Autodesk Inventor part; units mm, degrees
ref_plane "YZ Plane" through (0, 0, 0) normal (1, 0, 0) x (0, 1, 0)
ref_plane "XZ Plane" through (0, 0, 0) normal (0, 1, 0) x (-1, 0, 0)
ref_plane "XY Plane" through (0, 0, 0) normal (0, 0, 1) x (1, 0, 0)
sketch "Sketch1" plane through (0, 0, 0) normal (0, 0, 1) x (1, 0, 0)
  line L0 (-18.2958, -15.2546) -> (32.5042, -15.2546)
  line L1 (32.5042, -15.2546) -> (32.5042, 16.4954)
  line L2 (32.5042, 16.4954) -> (-18.2958, 16.4954)
  line L3 (-18.2958, 16.4954) -> (-18.2958, -15.2546)
  point P0 (0, 0)
  dimension "d0" = 50.8
  dimension "d1" = 31.75
extrude "Extrusion1" add sketch "Sketch1" along normal blind 31.75
sketch "Sketch2" plane through (0, 0, 31.75) normal (0, 0, 1) x (1, 0, 0)
  line L0 (32.5042, 16.4954) -> (-18.2958, 16.4954)
  line L1 (32.5042, -15.2546) -> (32.5042, 16.4954)
  line L2 (19.8042, 16.4954) -> (32.5042, 16.4954)
  line L3 (32.5042, 16.4954) -> (32.5042, 0.6204)
  line L4 (32.5042, 0.6204) -> (19.8042, 0.6204)
  line L5 (19.8042, 0.6204) -> (19.8042, 16.4954)
  line L6 (-18.2958, 16.4954) -> (-18.2958, -15.2546)
  line L7 (-18.2958, 0.6204) -> (-5.5958, 0.6204)
  line L8 (-5.5958, 0.6204) -> (-5.5958, 16.4954)
  line L9 (-5.5958, 16.4954) -> (-18.2958, 16.4954)
  line L10 (-18.2958, 16.4954) -> (-18.2958, 0.6204)
  point P0 (0, 0)
  dimension "d4" = 15.875
  dimension "d5" = 12.7
  dimension "d6" = 15.875
  dimension "d7" = 12.7
extrude "Extrusion2" cut sketch "Sketch2" against normal blind 31.75
sketch "Sketch3" plane through (0, 0, 31.75) normal (0, 0, 1) x (1, 0, 0)
  line L0 (-18.2958, -15.2546) -> (32.5042, -15.2546)
  line L1 (-11.9458, -15.2546) -> (26.1542, -15.2546)
  line L2 (26.1542, -15.2546) -> (26.1542, -8.9046)
  line L3 (26.1542, -8.9046) -> (-11.9458, -8.9046)
  line L4 (-11.9458, -8.9046) -> (-11.9458, -15.2546)
  line L5 (-18.2958, 0.6204) -> (-18.2958, -15.2546)
  line L6 (32.5042, -15.2546) -> (32.5042, 0.6204)
  point P0 (0, 0)
  dimension "d10" = 6.35
  dimension "d11" = 6.35
  dimension "d12" = 6.35
extrude "Extrusion3" cut sketch "Sketch3" against normal blind 31.75
properties part number "Figure 7_27_2"
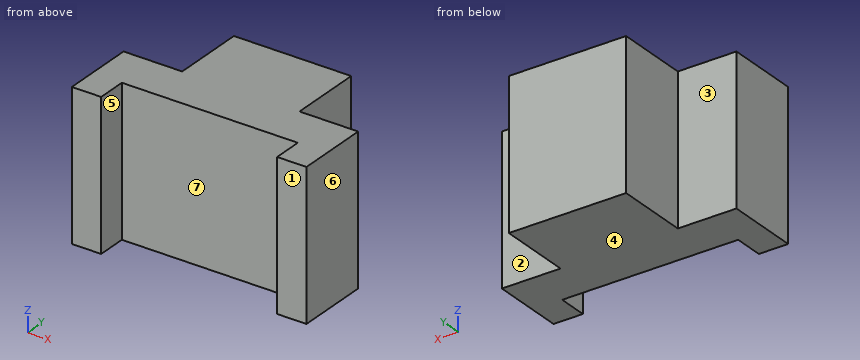
For this review, take the finished solid that the model builds, in its own axes (mm). Face numbers are marked on the shaded views. A direction names the side the tool comes from. Give positions to 0.01 mm unless a question says otherwise; leave off trailing zeros. Order: outer loops, then holes, each group sorted by start corner. A loop starts at its lowest first (then second) coordinate and runs counter-clockwise, first axis right, second up.
1) For the marked faces 1, 2 and 3, list the 3-axis set-ups (+Z, -Z, +X, -X, +Y, -Y) from which the entire face can be reached by the end or side of a thin tool; tool diameter is ignored.
2) Wall thickness on line 1 (X direction, y = -13, z = 24); line 2 (Y direction, x = 19, z = 26.5); line 3 (Y direction, x = 25, z = 10): over which ranges is each line inside the solid? List them lowest first.
3) Take a section at C-C (y = 2). Give the boundary of the cut face in (x, z).
4) Take a section at A-A (z = 24). Give the boundary of the cut face in (x, y), then the cut area to 3 significant figures.
5) Take a section at B-B (x = -13). Give the boundary of the cut face in (y, z).
6) Insertion check: pin 1 (4 mm diameter, centred on x = 29, z = 19.5, fed in from +Y); pin 2 (5 mm diameter, centred on y = 8.5, z = 18.5, fed in from -X); pin 3 (8 mm diameter, centred on y = 7.5, z = 8.5, fed in from +X). Each pin has a flat end and moves straight along its axis. Give the tip position at first contact, or say it passes through.
7) The part is to be moulded in two halves that separate along X. For the marked faces 4, 5, 6 and 7, say which applies: released by +X, released by -X, zero draft, split by the parting line, or undercut.
Derived:
1. face 1: +Z, -Z, +X, -X, -Y
1. face 2: +Z, -Z, +X, +Y
1. face 3: +Z, -Z, -X, +Y
2. line 1: x = -18.3 to -11.95, 26.15 to 32.5
2. line 2: y = -8.9 to 16.5
2. line 3: y = -8.9 to 0.62
3. outline: (-5.6, 0) - (19.8, 0) - (19.8, 31.75) - (-5.6, 31.75) - close
4. outline: (-18.3, -15.25) - (-11.95, -15.25) - (-11.95, -8.9) - (26.15, -8.9) - (26.15, -15.25) - (32.5, -15.25) - (32.5, 0.62) - (19.8, 0.62) - (19.8, 16.5) - (-5.6, 16.5) - (-5.6, 0.62) - (-18.3, 0.62) - close
4. area: 968 mm2
5. outline: (-15.25, 0) - (0.62, 0) - (0.62, 31.75) - (-15.25, 31.75) - close
6. pin 1: stops at y = 0.62
6. pin 2: stops at x = -5.6
6. pin 3: stops at x = 19.8
7. face 4: zero draft
7. face 5: undercut
7. face 6: released by +X
7. face 7: undercut
